```python
from build123d import *

# Parameters (mm, degrees)
F0_W     = 39.76
F0_H     = 42
F0_R     = 3.74
F0_R_2   = 6.55
F1_DEPTH = 8.1
F2_R     = 9.906
F2_R_2   = 6.55
F3_DEPTH = 13.14
F4_R     = 1


with BuildPart() as f1:
    # F0 (on Front) → F1 (new body, symmetric)
    with BuildSketch(Plane.XZ):
        with Locations((19.88, 21)):
            Rectangle(F0_W, F0_H)
        with Locations((19.88, 9.053554)):
            Circle(F0_R, mode=Mode.SUBTRACT)
        with Locations((19.88, 30.481216)):
            Circle(F0_R_2, mode=Mode.SUBTRACT)
    extrude(amount=F1_DEPTH, both=True)

    # F2 (on face) → F3 (cut)
    with BuildSketch(Plane(origin=(0, 8.1, 0), x_dir=(-1, 0, 0), z_dir=(0, 1, 0))):
        with Locations((-19.88, 30.481216)):
            Circle(F2_R)
        with Locations((-19.88, 30.481216)):
            Circle(F2_R_2, mode=Mode.SUBTRACT)
    extrude(amount=-F3_DEPTH, mode=Mode.SUBTRACT)

    # F4
    f4_edges = [f1.edges().sort_by_distance(p)[0] for p in [
        (19.88, -8.1, 42),
        (39.76, -8.1, 21),
        (19.88, -8.1, 0),
        (39.76, 0, 42),
        (0, 0, 42),
        (19.88, 8.1, 42),
        (39.76, 8.1, 21),
        (39.76, 0, 0),
        (0, -8.1, 21),
        (0, 8.1, 21),
        (19.88, 8.1, 0),
        (0, 0, 0),
    ]]
    fillet(f4_edges, radius=F4_R)


solid = f1.part
```
Verification items for the finished model (mm, model axes). A direction names the side the tool comes from. Coordinates: 2 decimals unless noted, no trailing zeros. Loops run counter-clockwise (first coordinate to the right, second up) from the corner with the lowest first, then second, coordinate; pieces in that order, holes last. Notation, with made-up numbers: (29, 16.25) -> (51, 16.25) arc R27 cw to (51, 36.25) -> close; hole circle Ø2 at (76, 26.25). An arc over 180 degrees is marked (long way). Answer in a Markdown table with one row per item.
1) Section check B-B (z = 33). Record the cut outline in (x, y).
The answers:
| item | result |
|---|---|
| outline | (0, -7.1) arc R1 ccw to (1, -8.1) -> (13.83, -8.1) -> (13.83, -5.04) -> (10.3, -5.04) -> (10.3, 8.1) -> (1, 8.1) arc R1 ccw to (0, 7.1) -> close; (25.93, -8.1) -> (38.76, -8.1) arc R1 ccw to (39.76, -7.1) -> (39.76, 7.1) arc R1 ccw to (38.76, 8.1) -> (29.46, 8.1) -> (29.46, -5.04) -> (25.93, -5.04) -> close |
2) Section check D-D (y = -1.75). Record the cut outline in (x, z).
The answers:
| item | result |
|---|---|
| outline | (0, 1) arc R1 ccw to (1, 0) -> (38.76, 0) arc R1 ccw to (39.76, 1) -> (39.76, 41) arc R1 ccw to (38.76, 42) -> (1, 42) arc R1 ccw to (0, 41) -> close; hole circle Ø19.81 at (19.88, 30.48); hole circle Ø7.48 at (19.88, 9.05) |
3) Section check A-A (x = 19.88). Record the cut outline in (y, z).
The answers:
| item | result |
|---|---|
| outline | (-8.1, 1) arc R1 ccw to (-7.1, 0) -> (7.1, 0) arc R1 ccw to (8.1, 1) -> (8.1, 5.31) -> (-8.1, 5.31) -> close; (-8.1, 12.79) -> (8.1, 12.79) -> (8.1, 20.58) -> (-5.04, 20.58) -> (-5.04, 23.93) -> (-8.1, 23.93) -> close; (-8.1, 37.03) -> (-5.04, 37.03) -> (-5.04, 40.39) -> (8.1, 40.39) -> (8.1, 41) arc R1 ccw to (7.1, 42) -> (-7.1, 42) arc R1 ccw to (-8.1, 41) -> close |
4) Draft check along Z on faces 1 (the face through (21.9, 0.1, 12.2)), 2 (the face through (39.459, -7.815, 21.28)), 3 (the face through (0.285, 0.099, 41.699)), 4 (the face through (20.144, 7.815, 0.301)). Enter one of: released by +Z, released by -Z, zero draft, split by the parting line, or undercut.
The answers:
| item | result |
|---|---|
| face 1 | undercut |
| face 2 | zero draft |
| face 3 | released by +Z |
| face 4 | released by -Z |
5) Access from +Z, -Z, +X, -X, +Y, -Y to the whole of each face (thin tool, end or side, straight path). Record for faces 5 (the face through (20.144, -7.815, 41.699)), 6 (the face through (13, -5.04, 28)).
The answers:
| item | result |
|---|---|
| face 5 | +Z, +X, -X, -Y |
| face 6 | +Y |
6) Scan lines: line 1 along Z through (x, y) = (19, 5.25); line 2 along X through (y, z) = (-6.25, 32); line 3 along X through (y, z) = (5, 11.5). Record each from-to range of solid material in increasing order. Write a range as from..to.
The answers:
| item | result |
|---|---|
| line 1 | z = 0..5.42, 12.69..20.61, 40.35..42 |
| line 2 | x = 0..13.51, 26.25..39.76 |
| line 3 | x = 0..17.05, 22.71..39.76 |
7) Section check C-C (x = 14.5). Record the cut outline in (y, z), and give its area (3 significant figures).
The answers:
| item | result |
|---|---|
| outline | (-8.1, 1) arc R1 ccw to (-7.1, 0) -> (7.1, 0) arc R1 ccw to (8.1, 1) -> (8.1, 22.16) -> (-5.04, 22.16) -> (-5.04, 26.75) -> (-8.1, 26.75) -> close; (-8.1, 34.22) -> (-5.04, 34.22) -> (-5.04, 38.8) -> (8.1, 38.8) -> (8.1, 41) arc R1 ccw to (7.1, 42) -> (-7.1, 42) arc R1 ccw to (-8.1, 41) -> close |
| area | 438 mm2 |
